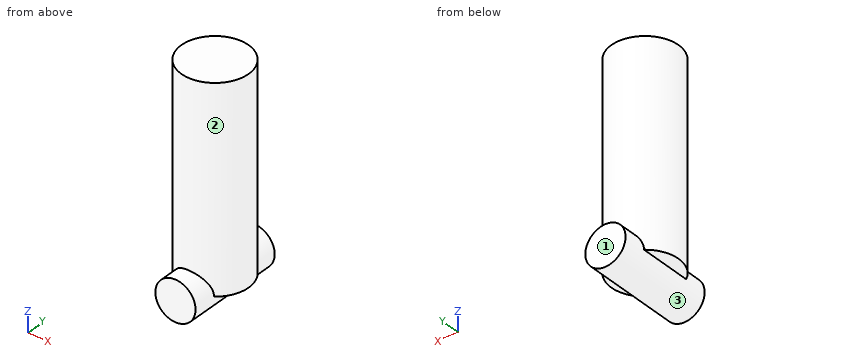
Autodesk Inventor part; units mm, degrees
sketch "スケッチ3" plane through (0, 0, 0) normal (0, 0, 1) x (1, 0, 0)
  circle A0 centre (0, 0) radius 25
  dimension "d7" = 50
extrude "押し出し2" add sketch "スケッチ3" against normal blind 200
sketch "スケッチ4" plane through (0, 0, 0) normal (0, 1, 0) x (-1, 0, 0)
  line L0 (50.5565, -50) -> (-56.0674, -50)
  line L1 (-56.0674, -50) -> (-56.0674, 47.5615)
  line L2 (-56.0674, 47.5615) -> (50.5565, 47.5615)
  line L3 (50.5565, 47.5615) -> (50.5565, -50)
  line L4 (-77.3922, 0) -> (71.8813, 0)
  point P0 (0, 0)
  dimension "d10" = 50
extrude "押し出し3" cut sketch "スケッチ4" along normal mid plane 200
sketch "スケッチ6" plane through (0, 0, 0) normal (0, 1, 0) x (-1, 0, 0)
  circle A0 centre (0, -200) radius 15
  line L0 (-35, 0) -> (35, 0)
  point P0 (0, 0)
  dimension "d13" = 30
  dimension "d14" = 200
extrude "押し出し4" add sketch "スケッチ6" along normal mid plane 75
properties part number "UpperarmY"
Model file for the job. Use its own axes, mm. Face numbers are marked on the shaded views. A direction names the side the tool comes from. Give positions to 0.01 mm unless a question says otherwise; leave off trailing zeros. Loops run counter-clockwise (first coordinate to the right, second up) from the corner with the lowest first, then second, coordinate; pieces in that order, holes last.
Item 1: Slice it at C-C (z = -101). Write the cut outline in (x, y).
Check values:
outline: circle Ø50 at (0, 0)
Item 2: Which spindle directions (+Z, -Z, +X, -X, +Y, -Y) get a long thin tool onto all of the face, cutting with end or side? Do the marked faces 1, 2 and 3. Say none if no direction does.
Check values:
face 1: +Z, -Z, +X, -X, +Y
face 2: +Z
face 3: none
Item 3: Slice it at B-B (y = 0). Write the cut outline in (x, z).
Check values:
outline: (-25, -200) - (-15, -200) arc R15 ccw to (15, -200) - (25, -200) - (25, -50) - (-25, -50) - close
Item 4: Drill centre lines: line 1 along Y through (x, z) = (0, -63); line 2 along Z through (x, y) = (18.5, 16); line 3 along Z through (x, y) = (1, 27.5). Where is each one in solid material? Low to high.
Check values:
line 1: y = -25 to 25
line 2: z = -200 to -50
line 3: z = -214.97 to -185.03
Item 5: Slice it at D-D (y = 29). Write the cut outline in (x, z), plus the area to 3 significant figures.
Check values:
outline: circle Ø30 at (0, -200)
area: 707 mm2
Item 6: Drop flat-ended pins along their axis: P1, Ø5, axis at y = -5.5, z = -67.5, coming from the -X side; P2, Ø8, axis at x = -19.5, y = 1.5, coming from the -Z side; P3, Ø1, axis at x = 10.5, z = -71, coming from the +Y side. Give the stop position or say it passes through.
Check values:
P1: stops at x = -24.82
P2: stops at z = -200
P3: stops at y = 22.91
Item 7: Slice it at A-A (x = 0). Write the cut outline in (y, z), plus the area to 3 significant figures.
Check values:
outline: (-37.5, -215) - (37.5, -215) - (37.5, -185) - (25, -185) - (25, -50) - (-25, -50) - (-25, -185) - (-37.5, -185) - close
area: 9,000 mm2
